Check sheet for the modelled part. Datum: model origin and axes. Units: mm. A direction names the side the tool comes from. Coordinates: 2 decimals unless noted, no trailing zeros. Loops run counter-clockwise (first coordinate to the right, second up) from the corner with the lowest first, then second, coordinate; pieces in that order, holes last.
from build123d import *

# Parameters (mm, degrees)
F1_DEPTH = 10
F2_R     = 2.5
F3_DEPTH = 25
F4_R     = 2.5
F5_DEPTH = 36.2


with BuildPart() as f1:
    # F0 (on Right) → F1 (new body)
    with BuildSketch(Plane.YZ):
        Polygon((-4, 0), (0, 0), (0, 23), (20, 23), (20, 27), (-4, 27), align=None)
    extrude(amount=F1_DEPTH)

    # F2 (on face) → F3 (cut)
    with BuildSketch(Plane(origin=(0, 0, 0), x_dir=(-1, 0, 0), z_dir=(0, 1, 0))):
        with Locations((-5.093283, 6.856344)):
            Circle(F2_R)
    extrude(amount=-F3_DEPTH, mode=Mode.SUBTRACT)

    # F4 (on face) → F5 (cut)
    with BuildSketch(Plane.XY.offset(27)):
        with Locations((5, 15.083956)):
            Circle(F4_R)
    extrude(amount=-F5_DEPTH, mode=Mode.SUBTRACT)


solid = f1.part
(1) Section check C-C, the plane y = 14.75. Enter the section's corners in (x, z).
(2) Section check D-D, the plane z = 25.25. Enter the section's corners in (x, y), plus the area to 3 significant figures.
(3) Draft check along X on faces 3 (the face through (2.784, -1.972, 5.899)), 4 (the face through (10, -1, 19)), 5 (the face through (5, 0, 11)). Enter one of: pulls with the +X half, pulls with the -X half, needs draft (parallel to the pull), parting line crosses it, or undercut.
(4) Section check A-A, the plane z = 5. Enter the section's corners in (x, y), plus the area to 3 significant figures.
(5) Set-up check for faces 1 (the face through (5, 10, 23)), 2 (the face through (5, -2, 0)): record each of +Z, -Z, +X, -X, +Y, -Y from which the full face is reachable in a straight line by a thin tool's end or side.
(6) Section check B-B, the plane x = 7. Enter the section's corners in (y, z).
(7) Gauge pin test, flat ends, axial feed: P1, Ø5, axis at x = 7.5, z = 11.5, coming from the +Y side; P2, Ø4.5, axis at x = 5.09, z = 6.86, coming from the +Y side; P3, Ø6, axis at x = 8.5, y = 9, coming from the -Z side. Record the tip position at first contact, or that the pin passes through.
(8) Scan lines: line 1 along Y through (x, z) = (5, 25.85); line 2 along Y through (x, z) = (1, 16); line 3 along Z through (x, y) = (7.5, 14). Record each from-to range of solid material in increasing order.
Determined:
1. outline: (0, 23) - (2.52, 23) - (2.52, 27) - (0, 27) - close; (7.48, 23) - (10, 23) - (10, 27) - (7.48, 27) - close
2. outline: (0, -4) - (10, -4) - (10, 20) - (0, 20) - close; hole circle Ø5 at (5, 15.08)
2. area: 220 mm2
3. face 3: undercut
3. face 4: pulls with the +X half
3. face 5: needs draft
4. outline: (0, -4) - (3.42, -4) - (3.42, 0) - (0, 0) - close; (6.77, -4) - (10, -4) - (10, 0) - (6.77, 0) - close
4. area: 26.6 mm2
5. face 1: -Z, +X, -X, +Y
5. face 2: -Z, +X, -X, +Y, -Y
6. outline: (-4, 0) - (0, 0) - (0, 5.24) - (-4, 5.24) - close; (-4, 8.47) - (0, 8.47) - (0, 23) - (13.58, 23) - (13.58, 27) - (-4, 27) - close; (16.58, 23) - (20, 23) - (20, 27) - (16.58, 27) - close
7. P1: stops at y = 0
7. P2: passes through
7. P3: stops at z = 23
8. line 1: y = -4 to 12.58, 17.58 to 20
8. line 2: y = -4 to 0
8. line 3: z = 23 to 27
